The drawing under review shows one solid part. Ordinate dimensions are in mm from its lowest x, y, z. A direction names the side the tool comes from. Round coordinates to 2 decimals unless told otherwise and drop trailing zeros. Order: outer loops, then holes, each group sorted by start corner. A loop starts at its lowest first (then second) coordinate and runs counter-clockwise, first axis right, second up. Notation, with made-up numbers: (7.25, 68) -> (41.25, 68) arc R23 cw to (41.25, 84) -> close; hole circle Ø3 at (42, 54.5). An arc over 180 degrees is marked (long way). Use a Markdown table: item, result. Add a question column.
1) Consider section C-C (z = 7.75). State the section outline as (x, y) points, plus the area to 3 significant figures.
2) Consider section A-A (x = 16). State the section outline as (y, z) points, plus the area to 3 significant figures.
3) Wall thickness on line 1 along Y through (x, z) = (16, 2.6); line 2 along X through (y, z) = (41, 2.9); line 3 along X through (y, z) = (12, 4): over which ranges is each line inside the solid? List them lowest first. Write a range as [from, to].
4) Draft analysis for pull direction Y (two halves, no side actions). For the marked faces 6, 7, 8 and 9, state which applies: pulls with the +Y half, pulls with the -Y half, needs draft (parallel to the pull), parting line crosses it, or undercut.
5) Consider section D-D (y = 27). State the section outline as (x, z) points.
6) Clearance check with flat-ended pins moving along their axes: P1, Ø4, axis at y = 14.5, z = 11.5, coming from the -X side (3 decimals); P2, Ø6, axis at y = 13, z = 4.5, coming from the +X side; P3, Ø1.2, axis at y = 5.5, z = 1.5, coming from the -X side. State where each tip first meets the part, or that it passes through.
7) Machinability: for the marked faces 1, 2, 3, 4 and 5, which of the approach directions +Z, -Z, +X, -X, +Y, -Y give a long, thin tool a straight path to every point of the face, cutting with its end or side? Answer none if there is none.
8) Consider section B-B (y = 41). State the section outline as (x, z) points.
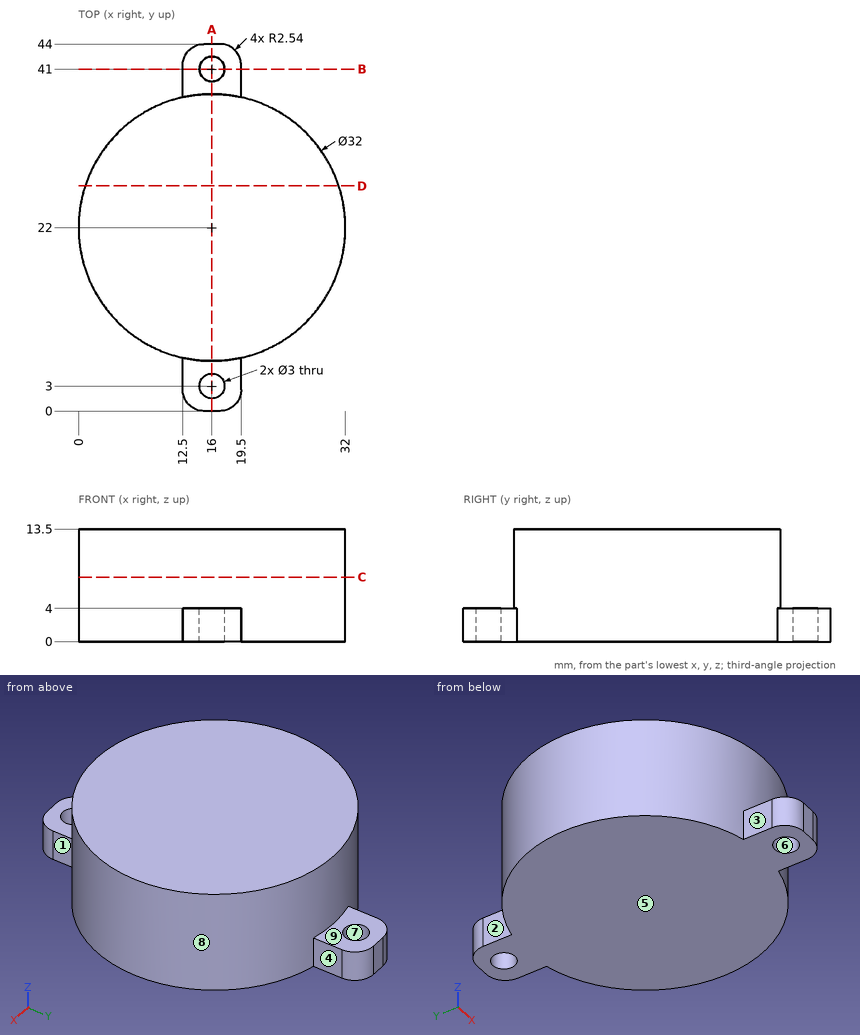
Results list:
| question | item | result |
|---|---|---|
| 1 | outline | circle Ø32 at (16, 22) |
| 1 | area | 804 mm2 |
| 2 | outline | (0, 0) -> (1.5, 0) -> (1.5, 4) -> (0, 4) -> close; (4.5, 0) -> (39.5, 0) -> (39.5, 4) -> (38, 4) -> (38, 13.5) -> (6, 13.5) -> (6, 4) -> (4.5, 4) -> close; (42.5, 0) -> (44, 0) -> (44, 4) -> (42.5, 4) -> close |
| 2 | area | 456 mm2 |
| 3 | line 1 | [0, 1.5], [4.5, 39.5], [42.5, 44] |
| 3 | line 2 | [12.5, 14.5], [17.5, 19.5] |
| 3 | line 3 | [3.51, 28.49] |
| 4 | face 6 | undercut |
| 4 | face 7 | undercut |
| 4 | face 8 | parting line crosses it |
| 4 | face 9 | needs draft |
| 5 | outline | (0.8, 0) -> (31.2, 0) -> (31.2, 13.5) -> (0.8, 13.5) -> close |
| 6 | P1 | x = 0.975 |
| 6 | P2 | x = 30.83 |
| 6 | P3 | x = 12.5 |
| 7 | face 1 | +Z, -Z, +X, -Y |
| 7 | face 2 | +Z, -Z, -X, +Y |
| 7 | face 3 | +Z, -Z, -X, -Y |
| 7 | face 4 | +Z, -Z, +X, +Y |
| 7 | face 5 | -Z, +X, -X, +Y, -Y |
| 8 | outline | (12.5, 0) -> (14.5, 0) -> (14.5, 4) -> (12.5, 4) -> close; (17.5, 0) -> (19.5, 0) -> (19.5, 4) -> (17.5, 4) -> close |
